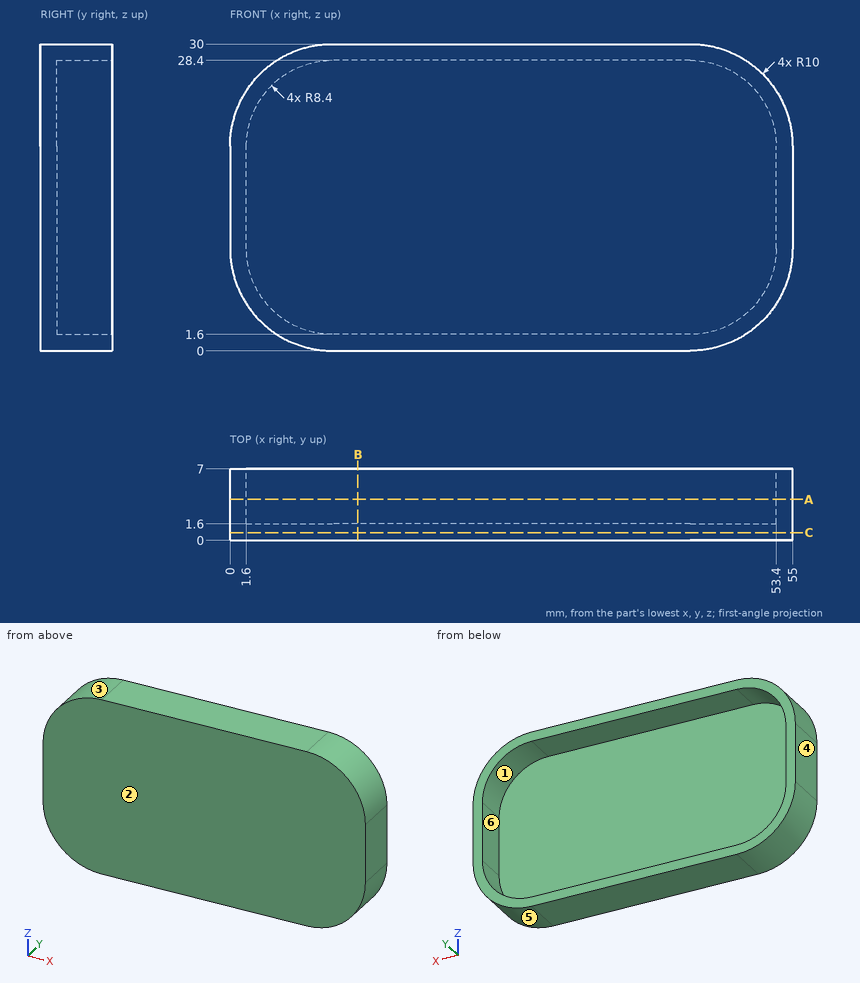
Geometry: see drawing. Coordinates: mm, zero at the bounding-box minimum. A direction names the side the tool comes from. Round coordinates to 2 decimals unless told otherwise and drop trailing zeros. Write each loop counter-clockwise with the first axis right and the second up, starting at its lowest first coordinate (ties: lowest second). Pieces come first, ordered by that corner, then holes. Notation, with made-up numbers: M 10,71.25 L 68,71.25 A11 cw 68,86.25 Z; hole C 39.25,5 d2. An arc over 180 degrees is marked long. Answer as a JSON object with one key per item and string values. Group by question number.
(1) Mould query, pull axis Z, two halves, no side actions, for the marked faces 3, 4, 5 and 6. Classes: +Z half, -Z half, draft (parallel to the pull), parting line (faces both ways), or undercut.
(2) Section query B-B on x = 12.5. Output: boundary loops of the cut face in (y, z).
(3) First-contact query: pin 1 (1 mm diameter, centred on y = 3.5, z = 23.5, fed in from -X); pin 2 (3 mm diameter, centred on y = 2.5, z = 25.5, fed in from -X); pin 3 (1 mm diameter, centred on x = 15, z = 13, fed in from +Y). Flat tips, straight axial feed; report the tip coordinate or a pass-through.
(4) Section query C-C on y = 0.75. Output: boundary loops of the cut face in (x, z), then the cut area to 3 significant figures.
(5) Section query A-A on y = 4. Output: boundary loops of the cut face in (x, z), then the cut area to 3 significant figures.
(6) Reachability of the marked faces 1 and 2 from +Z, -Z, +X, -X, +Y, -Y: full face, straight path, thin tool, end or side. Return the list, or none.
(7) Ray query, line 1 (X direction, y = 2, z = 16); line 2 (Z direction, x = 35.5, y = 2.5); line 3 (Y direction, x = 25, z = 26). Return the intervals inside material, ascending. Write a range as [from, to].
Computed values:
{
 "1": {"face 3": "+Z half", "face 4": "draft", "face 5": "-Z half", "face 6": "undercut"},
 "2": {"outline": "M 0,0 L 7,0 L 7,1.6 L 1.6,1.6 L 1.6,28.4 L 7,28.4 L 7,30 L 0,30 Z"},
 "3": {"pin 1": "x = 0.46", "pin 2": "x = 0.83", "pin 3": "y = 1.6"},
 "4": {"outline": "M 0,10 A10 ccw 10,0 L 45,0 A10 ccw 55,10 L 55,20 A10 ccw 45,30 L 10,30 A10 ccw 0,20 Z", "area": "1,560 mm^2"},
 "5": {"outline": "M 0,10 A10 ccw 10,0 L 45,0 A10 ccw 55,10 L 55,20 A10 ccw 45,30 L 10,30 A10 ccw 0,20 Z; hole M 1.6,10 A8.4 ccw 10,1.6 L 45,1.6 A8.4 ccw 53.4,10 L 53.4,20 A8.4 ccw 45,28.4 L 10,28.4 A8.4 ccw 1.6,20 Z", "area": "236 mm^2"},
 "6": {"face 1": "+Y", "face 2": "+Z, -Z, +X, -X, -Y"},
 "7": {"line 1": "[0, 1.6], [53.4, 55]", "line 2": "[0, 1.6], [28.4, 30]", "line 3": "[0, 1.6]"}
}
